Check sheet for the modelled part. Datum: model origin and axes. Units: mm. Coordinates: 2 decimals unless noted, no trailing zeros. Loops run counter-clockwise (first coordinate to the right, second up) from the corner with the lowest first, then second, coordinate; pieces in that order, holes last. Notation, with made-up numbers: (-40, 9) -> (-22, 9) arc R27 ccw to (-22, 29) -> close; hole circle Ø9 at (21.5, 88.25). An arc over 180 degrees is marked (long way). Use CSV: the item, a comma, the result in double quotes. Start each with the question number.
1. Sectioned sample at A-A, the plane z = 30.5. Record the cut outline in (x, y).
2. Sectioned sample at B-B, the plane x = 47.25. Record the cut outline in (y, z).
3. Thickness scan on L1, parallel to X at y = 0.6, z = 30.5; L2, parallel to X at y = 1.85, z = 40.5; L3, parallel to Z at x = -73.5, y = 0.25. Record the ranges inside material, lowest first.
4. Gauge pin test, flat ends, axial feed: pin 1 (0.8 mm diameter, centred on x = 40, y = 0.5, fed in from -Z); pin 2 (3 mm diameter, centred on x = 47.25, z = 40.5, fed in from +Y); pin 3 (0.5 mm diameter, centred on y = 0.5, z = -14.5, fed in from -X); pin 4 (0.8 mm diameter, centred on x = -30, y = 0.5, fed in from +Z). Record the tip position at first contact, or that the pin passes through.
5. Sectioned sample at C-C, the plane x = -46.5. Record the cut outline in (y, z).
6. Sectioned sample at D-D, the plane z = -58. Record the cut outline in (x, y).
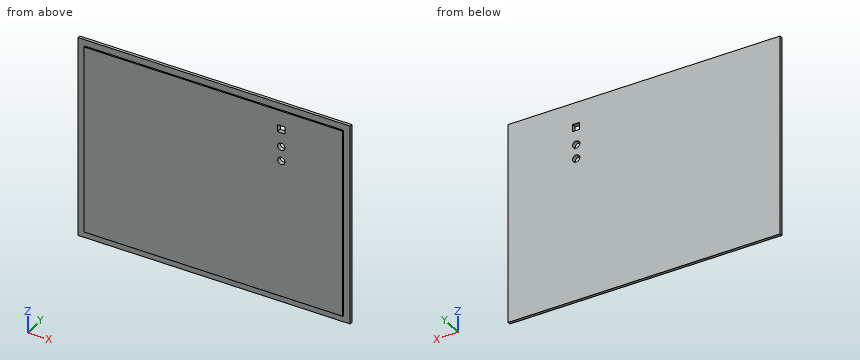
```python
from build123d import *

# Parameters (mm, degrees)
ESBO_O1_W                = 179.9
ESBO_O1_H                = 131.9
RESSALTO_EXTRUS_O1_DEPTH = 1
ESBO_O2_W                = 189
ESBO_O2_H                = 141
RESSALTO_EXTRUS_O2_DEPTH = 2
ESBO_O3_R                = 2.55
ESBO_O3_W                = 5
ESBO_O3_H                = 5
CORTE_EXTRUS_O1_DEPTH    = 118.938543318


with BuildPart() as part:
    # Esboço1 → Ressalto-extrusão1 (new body)
    with BuildSketch(Plane(origin=(0, 0, 0), x_dir=(1, 0, 0), z_dir=(0, 1, 0))):
        Rectangle(ESBO_O1_W, ESBO_O1_H)
    extrude(amount=RESSALTO_EXTRUS_O1_DEPTH)

    # Esboço2 → Ressalto-extrusão2 (add)
    with BuildSketch(Plane(origin=(0, 1, 0), x_dir=(1, 0, 0), z_dir=(0, 1, 0))):
        Rectangle(ESBO_O2_W, ESBO_O2_H)
    extrude(amount=RESSALTO_EXTRUS_O2_DEPTH)

    # Esboço3 → Corte-extrusão1 (cut, through all)
    with BuildSketch(Plane(origin=(0, 3, 0), x_dir=(1, 0, 0), z_dir=(0, 1, 0))):
        with Locations(Location((47.25, -40.5, 0), (0, 0, 270))):
            Circle(ESBO_O3_R)
        with Locations(Location((47.25, -30.5, 0), (0, 0, 270))):
            Circle(ESBO_O3_R)
        with Locations((47.25, -53)):
            Rectangle(ESBO_O3_W, ESBO_O3_H)
    extrude(amount=-CORTE_EXTRUS_O1_DEPTH, mode=Mode.SUBTRACT)


solid = part.part
```
Completed:
1,outline,"(-94.5, 1) -> (-89.95, 1) -> (-89.95, 0) -> (44.7, 0) -> (44.7, 3) -> (-94.5, 3) -> close; (49.8, 0) -> (89.95, 0) -> (89.95, 1) -> (94.5, 1) -> (94.5, 3) -> (49.8, 3) -> close"
2,outline,"(0, -65.95) -> (1, -65.95) -> (1, -70.5) -> (3, -70.5) -> (3, 27.95) -> (0, 27.95) -> close; (0, 33.05) -> (3, 33.05) -> (3, 37.95) -> (0, 37.95) -> close; (0, 43.05) -> (3, 43.05) -> (3, 50.5) -> (0, 50.5) -> close; (0, 55.5) -> (3, 55.5) -> (3, 70.5) -> (1, 70.5) -> (1, 65.95) -> (0, 65.95) -> close"
3,L1,"-89.95 to 44.7, 49.8 to 89.95"
3,L2,"-94.5 to 44.7, 49.8 to 94.5"
3,L3,"-65.95 to 65.95"
4,pin 1,"z = -65.95"
4,pin 2,"through"
4,pin 3,"x = -89.95"
4,pin 4,"z = 65.95"
5,outline,"(0, -65.95) -> (1, -65.95) -> (1, -70.5) -> (3, -70.5) -> (3, 70.5) -> (1, 70.5) -> (1, 65.95) -> (0, 65.95) -> close"
6,outline,"(-94.5, 1) -> (-89.95, 1) -> (-89.95, 0) -> (89.95, 0) -> (89.95, 1) -> (94.5, 1) -> (94.5, 3) -> (-94.5, 3) -> close"
